Autodesk Inventor part; units mm, degrees
ref_plane "Plano de trabajo1" through (54.9878, 17.2439, -20.5971) normal (1, 0, 0) x (0, 0, -1)
ref_plane "Plano de trabajo3" through (27.4939, 50, 0) normal (1, 0, 0) x (0, -1, 0)
ref_plane "Plano de trabajo6" through (46.7808, 33.3843, -20.5971) normal (-1, 0, 0) x (0, 0, 1)
sketch "Boceto1" plane through (0, 0, 0) normal (0, 1, 0) x (-1, 0, 0)
  circle A0 centre (0, 0) radius 10
  line L0 (-4.9878, -8.6673) -> (-54.9878, -8.6673)
  line L1 (-6.7993, 7.3327) -> (-53.4848, 7.3327)
  line L2 (-54.9878, -8.6673) -> (-87.1955, 1.2044)
  arc A1 (-81.3346, 20.3264) -> (-87.1955, 1.2044) centre (-84.2651, 10.7654) ccw
  line L3 (-81.3346, 20.3264) -> (-53.4848, 7.3327)
  dimension "d0" = 20
  dimension "d1" = 16
  dimension "d2" = 10
  dimension "d3" = 50
  dimension "d25" = 154.988
extrude "Extrusión1" add sketch "Boceto1" along normal blind 50
sketch "Boceto2" plane through (54.9878, 0, -8.6673) normal (0, 0, -1) x (-1, 0, 0)
  line L0 (-39.2772, 0) -> (-39.2772, 50)
  line L1 (-32.2077, 50) -> (0, 50)
  line L2 (-32.2077, 0) -> (0, 0)
  line L3 (0, 0) -> (50, 0)
  line L4 (0, 50) -> (50, 50)
  line L5 (92.4078, 25) -> (-89.4019, 25)
  line L6 (-39.2772, 17) -> (-18.1038, 17)
  line L7 (-16.1038, 19) -> (-16.1038, 25)
  line L8 (-39.2772, 13) -> (-9.2772, 13)
  line L9 (-9.2772, 13) -> (20, 0)
  line L10 (48.1885, 0) -> (1.503, 0)
  line L11 (8.207, 25) -> (8.207, 17.2439)
  line L12 (9.1152, 15.5682) -> (17.5023, 10.1036)
  line L13 (18.5941, 9.7793) -> (44, 9.7793)
  line L14 (46, 11.7793) -> (46, 25)
  line L15 (50, 0) -> (20, 0)
  line L16 (64.9878, 0) -> (48.1885, 0)
  line L17 (50, 50) -> (50, 0)
  arc A0 (-18.1038, 17) -> (-16.1038, 19) centre (-18.1038, 19) ccw
  arc A1 (8.207, 17.2439) -> (9.1152, 15.5682) centre (10.207, 17.2439) ccw
  arc A2 (17.5023, 10.1036) -> (18.5941, 9.7793) centre (18.5941, 11.7793) ccw
  arc A3 (44, 9.7793) -> (46, 11.7793) centre (44, 11.7793) ccw
  line L18 (20, 0) -> (-39.2772, 0)
  line L19 (-26.3468, 0) -> (-39.2772, 0)
  line L20 (-39.2772, 17) -> (-39.2772, 25)
  line L21 (0, 50) -> (50, 50)
  line L22 (-39.2772, 33) -> (-18.1038, 33)
  line L23 (-16.1038, 31) -> (-16.1038, 25)
  line L24 (-39.2772, 37) -> (-9.2772, 37)
  line L25 (-9.2772, 37) -> (20, 50)
  line L26 (48.1885, 50) -> (1.503, 50)
  line L27 (8.207, 25) -> (8.207, 32.7561)
  line L28 (9.1152, 34.4318) -> (17.5023, 39.8964)
  line L29 (18.5941, 40.2207) -> (44, 40.2207)
  line L30 (46, 38.2207) -> (46, 25)
  line L31 (50, 0) -> (50, 50)
  arc A4 (-16.1038, 31) -> (-18.1038, 33) centre (-18.1038, 31) ccw
  arc A5 (9.1152, 34.4318) -> (8.207, 32.7561) centre (10.207, 32.7561) ccw
  arc A6 (18.5941, 40.2207) -> (17.5023, 39.8964) centre (18.5941, 38.2207) ccw
  arc A7 (46, 38.2207) -> (44, 40.2207) centre (44, 38.2207) ccw
  line L32 (20, 50) -> (-39.2772, 50)
  line L33 (-39.2772, 50) -> (-39.2772, 37)
  line L34 (-39.2772, 33) -> (-39.2772, 17)
  line L35 (-39.2772, 13) -> (-39.2772, 0)
  point P0 (54.9878, 0)
  point P1 (1.503, 25)
  point P2 (18, 9.7793)
  point P3 (46, 9.7793)
  dimension "d6" = 12
  dimension "d7" = 4
  dimension "d8" = 30
  dimension "d9" = 30
  dimension "d10" = 28
  dimension "d11" = 4
  dimension "d12" = 2
extrude "Extrusión2" cut sketch "Boceto2" against normal through all contours L0 L8 L9 L3 L2 L18 | L0 L5 L7 A0 L6 | L0 L22 A4 L23 L5 | L0 L32 L1 L4 L25 L24 | L27 A5 L28 A6 L29 A7 L30 L5 | L5 L14 A3 L13 A2 L12 A1 L11
sketch "Boceto3" plane through (0, 50, 0) normal (0, 1, 0) x (1, 0, 0)
  circle A0 centre (0, 0) radius 5
  arc A1 (81.3346, -20.3264) -> (87.1955, -1.2044) centre (84.2651, -10.7654) ccw
  circle A2 centre (84.2651, -10.7654) radius 3
  dimension "d15" = 10
  dimension "d16" = 6
extrude "Extrusión3" cut sketch "Boceto3" against normal through all
sketch "Boceto4" plane through (4.9878, 0, -8.6673) normal (0, 0, -1) x (-1, 0, 0)
  line L0 (-50, 8.8806) -> (-50, 41.1194)
  line L1 (-41.793, 17.2439) -> (-50, 17.2439)
  line L2 (-50, 17.2439) -> (-50, 33.3843)
  line L3 (-50, 33.3843) -> (-41.793, 33.3843)
  line L4 (-41.793, 33.3843) -> (-41.793, 17.2439)
  point P0 (4.9878, 0)
extrude "Extrusión4" add sketch "Boceto4" along normal blind 20
sketch "Boceto5" plane through (54.9878, 17.2439, -8.6673) normal (1, 0, 0) x (0, 0, -1)
  line L0 (20, 16.1404) -> (20, 0)
  line L1 (0, 16.1404) -> (20, 16.1404)
  line L2 (0, 0) -> (20, 0)
  circle A0 centre (11.9298, 8.0702) radius 8.0702
  line L3 (11.9298, 16.1404) -> (20, 16.1404)
  line L4 (20, 16.1404) -> (20, 8.0702)
  line L5 (20, 8.0702) -> (20, 0)
  line L6 (20, 0) -> (11.9298, 0)
  circle A1 centre (11.9298, 8.0702) radius 4
  point P0 (-8.6673, -17.2439)
  dimension "d21" = 8
extrude "Extrusión5" cut sketch "Boceto5" against normal up to next contours L0 A0 L1 | L0 L2 A0 | A1
ref_plane "Plano de trabajo1" through (54.9878, 17.2439, -20.5971) normal (1, 0, 0) x (0, 0, -1)
ref_plane "Plano de trabajo3" through (27.4939, 50, 0) normal (1, 0, 0) x (0, -1, 0)
ref_plane "Plano de trabajo2" through (0, 50, 0) normal (1, 0, 0) x (0, -1, 0)
mirror "Simetría1" about plane through (27.4939, 50, 0) normal (1, 0, 0) of "Extrusión5", "Extrusión4"
ref_plane "Plano de trabajo6" through (46.7808, 33.3843, -20.5971) normal (-1, 0, 0) x (0, 0, 1)
properties part number "wheel_holder" material "Acero inoxidable, austenítico"
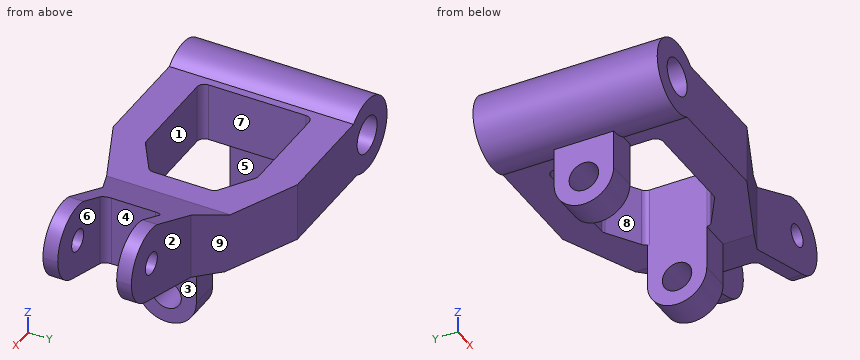
Can you work these out from the model? Positions are in its coordinate system, mm. Face numbers are marked on the shaded views. A direction names the side the tool comes from. Round coordinates to 2 decimals unless told otherwise and drop trailing zeros. Order: outer loops, then holes, each group sorted by start corner. A loop starts at its lowest first (then second) coordinate and runs counter-clockwise, first axis right, second up. Notation, with made-up numbers: M 5.25,88.5 L 33.25,88.5 A9 cw 33.25,93.5 Z; hole C 24,70.25 d10. An arc over 180 degrees is marked long. Use a Markdown table: item, result.
1) Imagine slicing it at B-B (x = 76). List the corners of the cut face in (y, z) for me, then the cut area to 3 significant figures.
Geometry says:
| item | result |
|---|---|
| outline | M 13,-2.23 L 17,-2.23 L 17,17.84 L 13,17.84 Z; M 33,-2.23 L 37,-2.23 L 37,17.84 L 33,17.84 Z |
| area | 161 mm² |
2) If we mould it in two halves opening along X, with no side actions, what happens to the marked faces 6, 7, 8 and 9? For each: +X half, -X half, draft (parallel to the pull), parting line (faces both ways), or undercut.
Geometry says:
| item | result |
|---|---|
| face 6 | draft |
| face 7 | undercut |
| face 8 | undercut |
| face 9 | +X half |
3) On a 3-axis mill with a long thin cutter (end or side, diameter ignored), from which of +Z, -Z, +X, -X, +Y, -Y can I reach the whole of each face in a straight line? I mean the marked faces 1, 2, 3, 4 and 5. Say none if no direction works.
Geometry says:
| item | result |
|---|---|
| face 1 | +Z, -Z |
| face 2 | +Z, -Z, +X, +Y |
| face 3 | -Z, +X, +Y, -Y |
| face 4 | +Z, -Z, +X |
| face 5 | -Z, +Y, -Y |
4) I'm going to push flat-ended pins straight in: P1, Ø2, axis at y = 19, z = 7, coming from the -X side; P2, Ø7, axis at y = 25.31, z = -20.6, coming from the -X side; P3, Ø25, axis at x = 29, y = 35.5, coming from the -Z side; P4, Ø13, axis at y = 25.31, z = -20.6, coming from the +X side. Where does each tip first touch, or does it pass through?
Geometry says:
| item | result |
|---|---|
| P1 | stops at x = -8 |
| P2 | passes through |
| P3 | stops at z = -8.67 |
| P4 | stops at x = 54.99 |
5) Imagine slicing it at D-D (y = 4). List the corners of the cut face in (x, z) for me, then the cut area to 3 significant figures.
Geometry says:
| item | result |
|---|---|
| outline | M 4.99,-8.67 L 44,-8.67 L 44,7.33 L 6.8,7.33 A10 ccw long Z; hole C 0,0 d10 |
| area | 799 mm² |
6) Imagine slicing it at A-A (z = 0). Give the number of separate pieces and of enclosed holes in the cut face, then the cut area to 3 significant figures.
Geometry says:
| item | result |
|---|---|
| separate pieces | 2 |
| enclosed holes | 1 |
| area | 2,010 mm² |
7) Imagine slicing it at C-C (z = -19.5). List the corners of the cut face in (x, y) for me, then the cut area to 3 significant figures.
Geometry says:
| item | result |
|---|---|
| outline | M 0,17.24 L 8.21,17.24 L 8.21,21.47 L 0,21.47 Z; M 0,29.16 L 8.21,29.16 L 8.21,33.38 L 0,33.38 Z; M 46.78,17.24 L 54.99,17.24 L 54.99,21.47 L 46.78,21.47 Z; M 46.78,29.16 L 54.99,29.16 L 54.99,33.38 L 46.78,33.38 Z |
| area | 139 mm² |
8) If I drill on line 1 along X through (y, z) = (21.5, -23); line 2 along Y through (x, z) = (19.5, 3); line 3 along Y through (x, z) = (68.5, 14), over which ranges is the centre line in solid material (lowest first)?
Geometry says:
| item | result |
|---|---|
| line 1 | x = 0 to 8.21, 46.78 to 54.99 |
| line 2 | y = 0 to 9.78, 40.22 to 50 |
| line 3 | y = 13 to 37 |
